from build123d import *

# Parameters (mm, degrees)
SKETCH_1_W          = 10
SKETCH_1_H          = 180
EXTRUDE_1_DEPTH     = 30
SKETCH_3_R          = 5
CUT_EXTRUDE_3_DEPTH = 30


with BuildPart() as part:
    # Эскиз1 → Бобышка-Вытянуть1 (new body)
    with BuildSketch(Plane(origin=(0, 0, 0), x_dir=(1, 0, 0), z_dir=(0, 1, 0))):
        with Locations((32.217123935, 54.617723996)):
            Rectangle(SKETCH_1_W, SKETCH_1_H)
    extrude(amount=EXTRUDE_1_DEPTH)

    # Эскиз3 → Вырез-Вытянуть3 (cut)
    with BuildSketch(Plane(origin=(37.217123935, 0, 0), x_dir=(0, 0, -1), z_dir=(1, 0, 0))):
        with BuildLine():
            ThreePointArc((129.617723996, 30), (140.224325714, 25.606601718), (144.617723996, 15))
            Line((144.617723996, 15), (144.617723996, 30))
            Line((144.617723996, 30), (129.617723996, 30))
        make_face()
        with BuildLine():
            Line((129.617723996, 0), (144.617723996, 0))
            Line((144.617723996, 0), (144.617723996, 15))
            ThreePointArc((144.617723996, 15), (140.224325714, 4.393398282), (129.617723996, 0))
        make_face()
        with BuildLine():
            Line((-35.382276004, 0), (-20.382276004, 0))
            ThreePointArc((-20.382276004, 0), (-30.988877721, 4.393398282), (-35.382276004, 15))
            Line((-35.382276004, 15), (-35.382276004, 0))
        make_face()
        with BuildLine():
            ThreePointArc((-35.382276004, 15), (-30.988877721, 25.606601718), (-20.382276004, 30))
            Line((-20.382276004, 30), (-35.382276004, 30))
            Line((-35.382276004, 30), (-35.382276004, 15))
        make_face()
        with Locations((129.617723996, 15)):
            Circle(SKETCH_3_R)
        with Locations((-20.382276004, 15)):
            Circle(SKETCH_3_R)
    extrude(amount=-CUT_EXTRUDE_3_DEPTH, mode=Mode.SUBTRACT)


solid = part.part
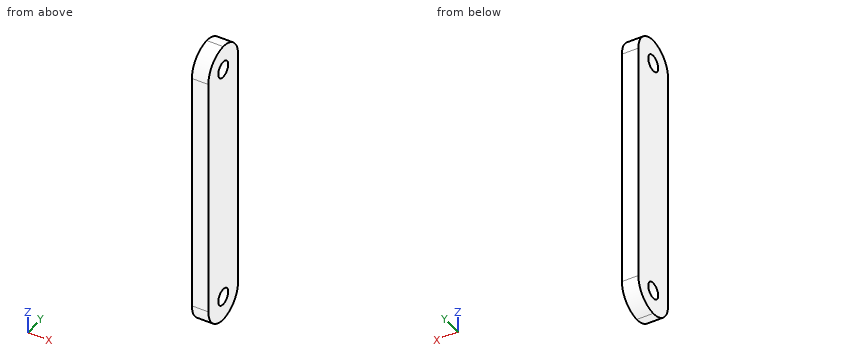
The listing builds one solid part. Answer for the finished solid, in the listing's coordinates (mm). Give positions to 0.01 mm unless a question says otherwise; leave off trailing zeros. Order: outer loops, then holes, each group sorted by start corner. A loop starts at its lowest first (then second) coordinate and runs counter-clockwise, first axis right, second up. Notation, with made-up numbers: (44, -34.5) - (96, -34.5) arc R9 cw to (96, -27.5) - close; hole circle Ø3 at (-26, 48.5). An arc over 180 degrees is marked (long way). Use one line per item in the form item = value.
1) Consider probe 1 along Z at (x, y) = (33.5, 16); probe 2 along Y at (x, z) = (30.25, -128.5); probe 3 along Y at (x, z) = (32, 22.5). Determine where each line is inside the solid, lowest interval first. Write a range as [from, to].
Verdict:
probe_1 = [-144.58, -134.52], [-124.72, 15.48], [25.28, 35.35]
probe_2 = [0, 10.13], [19.87, 30]
probe_3 = [0.15, 10.47], [19.53, 29.85]
2) Each of these flat-tipped pins is pushed along its axis until it touches: pin 1 (6 mm diameter, centred on y = 15, z = 20.38, fed in from -X); pin 2 (4 mm diameter, centred on x = 34, y = 25, fed in from -Z); pin 3 (3 mm diameter, centred on x = 29.5, y = 17, fed in from -Z); pin 4 (2 mm diameter, centred on x = 33.5, y = 23.5, fed in from +Z). Where does it stop, or does it pass through?
Verdict:
pin_1 = through
pin_2 = -142.31
pin_3 = -144.61
pin_4 = 33.37
3) Find section C-C on y = 7. Determine the outline of the cut face in (x, z).
Verdict:
outline = (27.22, -142.31) - (37.22, -142.31) - (37.22, 33.07) - (27.22, 33.07) - close
4) Find section B-B on y = 22. Determine the outline of the cut face in (x, z).
Verdict:
outline = (27.22, -142.88) - (37.22, -142.88) - (37.22, 33.65) - (27.22, 33.65) - close
5) Find section A-A on x = 30.25. Determine the outline of the cut face in (y, z).
Verdict:
outline = (0, -129.62) arc R15 ccw to (30, -129.62) - (30, 20.38) arc R15 ccw to (0, 20.38) - close; hole circle Ø10 at (15, -129.62); hole circle Ø10 at (15, 20.38)
